Design review of the part built by this model. Coordinates are the model's own, in mm. A direction names the side the tool comes from. Coordinates: 2 decimals unless noted, no trailing zeros. Write each loop counter-clockwise with the first axis right and the second up, starting at its lowest first coordinate (ties: lowest second). Pieces come first, ordered by that corner, then holes.
Q1. Machinability: for faces 1 (the face through (10, 37, -98)), 2 (the face through (46, 38, -44)), 3 (the face through (45, 16, -117.409)), which of the approach directions +Z, -Z, +X, -X, +Y, -Y give a long, thin tool a straight path to every point of the face, cutting with its end or side? Answer none if there is none.
Q2. Add section A-A, the plane x = 29.5. Give the boundary of the cut face in (y, z), plus the area to 3 significant figures.
Q3. Add section C-C, the plane y = 26.5. Give the boundary of the cut face in (x, z).
Q4. To check wall thickness, follow probe 1 along Z at (x, y) = (74.5, 5); probe 2 along Z at (x, y) = (71, 34); probe 3 along X at (y, z) = (3, -88). State the ranges of each line that lie inside material, in increasing order.
Q5. Clearance check with flat-ended pins moving along their axes: pin 1 Ø0.6 at (y, z) = (39.5, -53.5) entering from +X; pin 2 Ø1.6 at (x, y) = (45, 39.5) entering from +Z; pin 3 Ø10 at (x, z) = (13, -57.5) entering from +Y; pin 4 Ø1.6 at (y, z) = (39, -42.5) entering from -X. State where each tip first meets the part, or that it passes through.
Q6. The part is to be moulded in two halves that separate along X. For faces 4 (the face through (0, 19, -61)), 5 (the face through (45, 19, 0)), 6 (the face through (92, 19, -61)), 7 (the face through (45, 37, -86)), say which applies: +X half, -X half, draft (parallel to the pull), parting line (faces both ways), or undercut.
Q7. Add section B-B, the plane z = -90.5. Give the boundary of the cut face in (x, y), plus the area to 3 significant figures.
Q8. Add section D-D, the plane x = 85. Give the boundary of the cut face in (y, z), plus the area to 3 significant figures.
from build123d import *

# Parameters (mm, degrees)
SKETCH1_W           = 92
SKETCH1_H           = 123
BOSS_EXTRUDE1_DEPTH = 40
SKETCH2_W           = 72
SKETCH2_H           = 24
CUT_EXTRUDE1_DEPTH  = 159.723029205
SKETCH3_W           = 69
SKETCH3_H           = 76
CUT_EXTRUDE2_DEPTH  = 2
SKETCH5_W           = 23
SKETCH5_H           = 1.5
CUT_EXTRUDE4_DEPTH  = 159.230844022
FILLET1_R           = 2
SHELL10_START       = 7
SHELL10_DEPTH       = 24
SKETCH8_W           = 83.82309106
SKETCH8_H           = 110.483157271
CUT_EXTRUDE6_DEPTH  = 33


# Read off the part's stored shape, not the designer's step: Shell10
with BuildPart() as part:
    # Sketch1 → Boss-Extrude1 (new body)
    with BuildSketch(Plane(origin=(0, 0, 0), x_dir=(1, 0, 0), z_dir=(0, 1, 0))):
        with Locations((46, 61.5)):
            Rectangle(SKETCH1_W, SKETCH1_H)
    extrude(amount=BOSS_EXTRUDE1_DEPTH)

    # Sketch2 → Cut-Extrude1 (cut, through all)
    with BuildSketch(Plane(origin=(0, 40, 0), x_dir=(1, 0, 0), z_dir=(0, 1, 0))):
        with Locations((46, 98)):
            Rectangle(SKETCH2_W, SKETCH2_H)
    extrude(amount=-CUT_EXTRUDE1_DEPTH, mode=Mode.SUBTRACT)

    # Sketch3 → Cut-Extrude2 (cut)
    with BuildSketch(Plane(origin=(0, 40, 0), x_dir=(1, 0, 0), z_dir=(0, 1, 0))):
        with Locations((46, 43)):
            Rectangle(SKETCH3_W, SKETCH3_H)
    extrude(amount=-CUT_EXTRUDE2_DEPTH, mode=Mode.SUBTRACT)

    # Sketch5 → Cut-Extrude4 (cut, through all)
    with BuildSketch(Plane(origin=(0, 38, 0), x_dir=(1, 0, 0), z_dir=(0, 1, 0))):
        with Locations((46, 10.75)):
            Rectangle(SKETCH5_W, SKETCH5_H)
    extrude(amount=-CUT_EXTRUDE4_DEPTH, mode=Mode.SUBTRACT)

    # Fillet1
    fillet1_edges = [part.edges().sort_by_distance(p)[0] for p in [
        (92, 40, -61.5),
        (46, 40, -123),
        (0, 40, -61.5),
        (0, 20, -123),
        (92, 20, -123),
        (92, 20, 0),
        (0, 20, 0),
        (46, 40, 0),
    ]]
    fillet(fillet1_edges, radius=FILLET1_R)

    # Shell10 outline → Shell10 (cut)
    with BuildSketch(Plane(origin=(0, 0, 0), x_dir=(1, 0, 0), z_dir=(0, 1, 0)).offset(SHELL10_START)):
        Polygon((7, 7), (27.5, 7), (27.5, 18.5), (64.5, 18.5), (64.5, 7), (85, 7), (85, 79), (7, 79), align=None)
    extrude(amount=SHELL10_DEPTH, mode=Mode.SUBTRACT)

    # Sketch8 → Cut-Extrude6 (cut)
    with BuildSketch(Plane.XZ):
        with Locations((45.787286948, -62.167007368)):
            Rectangle(SKETCH8_W, SKETCH8_H)
    extrude(amount=-CUT_EXTRUDE6_DEPTH, mode=Mode.SUBTRACT)


solid = part.part
Here are the results:
1. face 1: +Y, -Y
1. face 2: +Y
1. face 3: -Y
2. outline: (0, -123) - (38, -123) arc R2 ccw to (40, -121) - (40, -110) - (33, -110) - (33, -117.41) - (0, -117.41) - close; (0, -6.93) - (33, -6.93) - (33, -86) - (40, -86) - (40, -81) - (38, -81) - (38, -5) - (40, -5) - (40, -2) arc R2 ccw to (38, 0) - (0, 0) - close
2. area: 952 mm2
3. outline: (0, -121) arc R2 ccw to (2, -123) - (90, -123) arc R2 ccw to (92, -121) - (92, -2) arc R2 ccw to (90, 0) - (2, 0) arc R2 ccw to (0, -2) - close; hole (3.88, -117.41) - (87.7, -117.41) - (87.7, -6.93) - (3.88, -6.93) - close
4. probe 1: z = -123 to -117.41, -6.93 to 0
4. probe 2: z = -123 to -110, -86 to 0
4. probe 3: x = 0 to 3.88, 87.7 to 92
5. pin 1: stops at x = 91.6
5. pin 2: stops at z = -0.13
5. pin 3: stops at y = 40
5. pin 4: stops at x = 0.01
6. face 4: -X half
6. face 5: draft
6. face 6: +X half
6. face 7: undercut
7. outline: (0, 0) - (3.88, 0) - (3.88, 33) - (10, 33) - (10, 40) - (2, 40) arc R2 ccw to (0, 38) - close; (82, 33) - (87.7, 33) - (87.7, 0) - (92, 0) - (92, 38) arc R2 ccw to (90, 40) - (82, 40) - close
7. area: 408 mm2
8. outline: (0, -123) - (38, -123) arc R2 ccw to (40, -121) - (40, -2) arc R2 ccw to (38, 0) - (0, 0) - (0, -6.93) - (33, -6.93) - (33, -117.41) - (0, -117.41) - close
8. area: 1,270 mm2
